```python
from build123d import *

# Parameters (mm, degrees)
F0_W     = 8
F0_H     = 8
F0_R     = 3
F1_DEPTH = 2
F0_R_2   = 1.5
F2_DEPTH = 1


# Not quite as in the source:
# - a feature names something its author has since deleted; it is built from what else it names


with BuildPart() as f1:
    # F0 (on Top) → F1 (new body)
    with BuildSketch(Plane.XY):
        Polygon((4, -40.5), (75, -40.5), (75, -4), (67, -4), (67, 4), (75, 4), (75, 40.5), (4, 40.5), (4, 32.5), (-4, 32.5), (-4, 40.5), (-75, 40.5), (-75, 4), (-67, 4), (-67, -4), (-75, -4), (-75, -40.5), (-4, -40.5), (-4, -32.5), (4, -32.5), align=None)
        with Locations((-71, 0)):
            Rectangle(F0_W, F0_H)
        with Locations((-71, 0)):
            Circle(F0_R, mode=Mode.SUBTRACT)
        with Locations((0, 36.5)):
            Rectangle(F0_W, F0_H)
        with Locations((0, 36.5)):
            Circle(F0_R, mode=Mode.SUBTRACT)
        with Locations((71, 0)):
            Rectangle(F0_W, F0_H)
        with Locations((71, 0)):
            Circle(F0_R, mode=Mode.SUBTRACT)
        with Locations((0, -36.5)):
            Rectangle(F0_W, F0_H)
        with Locations((0, -36.5)):
            Circle(F0_R, mode=Mode.SUBTRACT)
    extrude(amount=F1_DEPTH)

    # F0 (on Top) → F2 (join)
    with BuildSketch(Plane.XY):
        with Locations((0, 36.5)):
            Circle(F0_R)
        with Locations((0, 36.5)):
            Circle(F0_R_2, mode=Mode.SUBTRACT)
        with Locations((71, 0)):
            Circle(F0_R)
        with Locations((71, 0)):
            Circle(F0_R_2, mode=Mode.SUBTRACT)
        with Locations((0, -36.5)):
            Circle(F0_R)
        with Locations((0, -36.5)):
            Circle(F0_R_2, mode=Mode.SUBTRACT)
        with Locations((-71, 0)):
            Circle(F0_R)
        with Locations((-71, 0)):
            Circle(F0_R_2, mode=Mode.SUBTRACT)
    extrude(amount=F2_DEPTH)


solid = f1.part
```
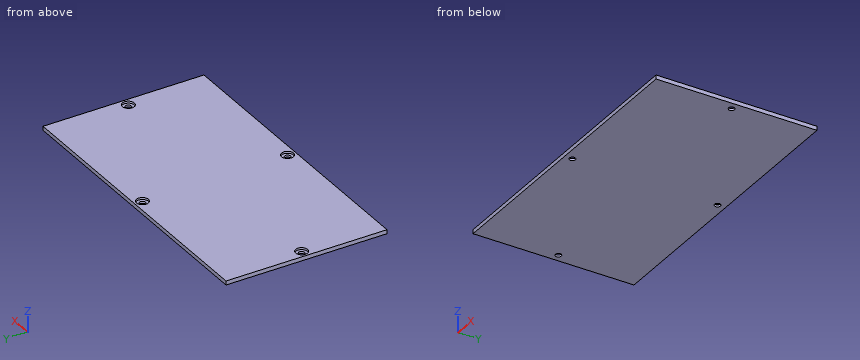
Build history of the part. All positions in model axes, mm. Round coordinates to 2 decimals unless told otherwise and drop trailing zeros. Write each loop counter-clockwise with the first axis right and the second up, starting at its lowest first coordinate (ties: lowest second). Pieces come first, ordered by that corner, then holes.
1) Band-saw the part on D-D, the plane x = 0. List the corners of the cut face in (y, z).
2) Band-saw the part on C-C, the plane y = 0. List the corners of the cut face in (x, z).
3) Drill centre lines: probe 1 along Y at (x, z) = (0, 1.75); probe 2 along Y at (x, z) = (-71, 0.45); probe 3 along Y at (x, z) = (71, 1.75). Where is each one in solid material? Low to high.
4) Pin check, flat tips, straight feed: pin 1 (5 mm diameter, centred on x = 0, y = 36.5, fed in from +Z); pin 2 (2.5 mm diameter, centred on x = 71, y = 0, fed in from -Z). Stop position of each tip, or through.
5) Band-saw the part on B-B, the plane y = 36.5. List the corners of the cut face in (x, z), and give its area (3 significant figures).
6) Band-saw the part on A-A, the plane x = -71. List the corners of the cut face in (y, z), and give its area (3 significant figures).
Ans:
1. outline: (-40.5, 0) - (-38, 0) - (-38, 1) - (-39.5, 1) - (-39.5, 2) - (-40.5, 2) - close; (-35, 0) - (35, 0) - (35, 1) - (33.5, 1) - (33.5, 2) - (-33.5, 2) - (-33.5, 1) - (-35, 1) - close; (38, 0) - (40.5, 0) - (40.5, 2) - (39.5, 2) - (39.5, 1) - (38, 1) - close
2. outline: (-75, 0) - (-72.5, 0) - (-72.5, 1) - (-74, 1) - (-74, 2) - (-75, 2) - close; (-69.5, 0) - (69.5, 0) - (69.5, 1) - (68, 1) - (68, 2) - (-68, 2) - (-68, 1) - (-69.5, 1) - close; (72.5, 0) - (75, 0) - (75, 2) - (74, 2) - (74, 1) - (72.5, 1) - close
3. probe 1: y = -40.5 to -39.5, -33.5 to 33.5, 39.5 to 40.5
3. probe 2: y = -40.5 to -1.5, 1.5 to 40.5
3. probe 3: y = -40.5 to -3, 3 to 40.5
4. pin 1: stops at z = 1
4. pin 2: passes through
5. outline: (-75, 0) - (-1.5, 0) - (-1.5, 1) - (-3, 1) - (-3, 2) - (-75, 2) - close; (1.5, 0) - (75, 0) - (75, 2) - (3, 2) - (3, 1) - (1.5, 1) - close
5. area: 291 mm2
6. outline: (-40.5, 0) - (-1.5, 0) - (-1.5, 1) - (-3, 1) - (-3, 2) - (-40.5, 2) - close; (1.5, 0) - (40.5, 0) - (40.5, 2) - (3, 2) - (3, 1) - (1.5, 1) - close
6. area: 153 mm2
